Work out the finished part from the listing and answer in its coordinate system (mm). Face numbers are marked on the shaded views. A direction names the side the tool comes from. Give positions to 0.01 mm unless a question says otherwise; leave off trailing zeros. Write each loop counter-clockwise with the first axis right and the second up, starting at its lowest first coordinate (ties: lowest second). Pieces come first, ordered by that corner, then holes. Notation, with made-up numbers: (25, 75) -> (76, 75) arc R23 ccw to (76, 111) -> close; hole circle Ø4 at (-29.75, 47.5). An arc over 180 degrees is marked (long way). Use a Markdown table: item, result. Add a question column.
Q1. Each of these flat-tipped pins is pushed along its axis until it touches: pin 1 Ø2.5 at (x, y) = (0.5, -5) entering from +Z; pin 2 Ø1.5 at (y, z) = (14, -2.5) entering from -X; pin 3 Ø0.8 at (y, z) = (-5, -1.5) entering from +X. Where does it stop, or does it pass through?
Q2. Section A-A, the plane y = -1.5 is taken. Give the vertices of the cut face in (x, z), plus the area to 3 significant figures.
Q3. Section B-B, the plane x = 0 is taken. Give the vertices of the cut face in (y, z), plus the area to 3 significant figures.
Q4. Section D-D, the plane y = 19.5 is taken. Give the vertices of the cut face in (x, z), plus the area to 3 significant figures.
Q5. Consider line 1 (Y direction, x = -3.5, z = -1.5); line 2 (Z direction, x = -4, y = 0.5); line 3 (Y direction, x = 0.5, z = 0.25). Determine where each line is inside the solid, lowest interval first.
Q6. For the marked faces 4, 5 and 6, determine the directions among +Z, -Z, +X, -X, +Y, -Y from which every point of the face is accessible in a straight line to the end or side of a thin tool.
Q7. Section C-C, the plane z = 0 is taken. Give the vertices of the cut face in (x, y).
Q8. For a pull along Y with two mould halves and no side action, classify the marked faces 1, 2 and 3 as pulls with the +Y half, pulls with the -Y half, needs draft (parallel to the pull), parting line crosses it, or undercut.
from build123d import *

# Parameters (mm, degrees)
ESQUISSE3_W        = 3
ESQUISSE3_H        = 1
BOSS_EXTRU_1_DEPTH = 8


with BuildPart() as part:
    # Esquisse1 → Révolution1 (revolve)
    with BuildSketch(Plane.XY):
        Polygon((0, 0), (-5, 0), (-5, 13), (-6, 13), (-6, 18), (-3, 18), (-3, 20.5), (0, 20.5), align=None)
    revolve(axis=Axis((0, 0, 0), (0, 1, 0)))

    # Esquisse2 → Révolution2 (revolve)
    with BuildSketch(Plane.XY):
        with BuildLine():
            Line((0, 20.5), (-5, 20.5))
            Line((-5, 20.5), (-5, 22.5))
            ThreePointArc((-5, 22.5), (-4.707106781, 23.207106781), (-4, 23.5))
            Line((-4, 23.5), (0, 23.5))
            Line((0, 23.5), (0, 20.5))
        make_face()
    revolve(axis=Axis((0, 20.5, 0), (0, 1, 0)))

    # Esquisse3 → Boss.-Extru.1 (add)
    with BuildSketch(Plane.XZ):
        with Locations((0, -1.5)):
            Rectangle(ESQUISSE3_W, ESQUISSE3_H)
        with Locations((0, 1.5)):
            Rectangle(ESQUISSE3_W, ESQUISSE3_H)
    extrude(amount=BOSS_EXTRU_1_DEPTH)


solid = part.part
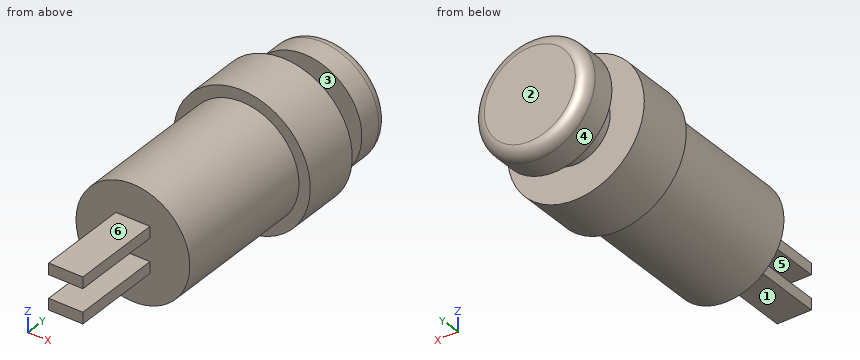
Result set:
| question | item | result |
|---|---|---|
| 1 | pin 1 | stops at z = 2 |
| 1 | pin 2 | stops at x = -5.74 |
| 1 | pin 3 | stops at x = 1.5 |
| 2 | outline | (-1.5, -2) -> (1.5, -2) -> (1.5, -1) -> (-1.5, -1) -> close; (-1.5, 1) -> (1.5, 1) -> (1.5, 2) -> (-1.5, 2) -> close |
| 2 | area | 6.00 mm2 |
| 3 | outline | (-8, -2) -> (0, -2) -> (0, -5) -> (13, -5) -> (13, -6) -> (18, -6) -> (18, -3) -> (20.5, -3) -> (20.5, -5) -> (22.5, -5) arc R1 ccw to (23.5, -4) -> (23.5, 4) arc R1 ccw to (22.5, 5) -> (20.5, 5) -> (20.5, 3) -> (18, 3) -> (18, 6) -> (13, 6) -> (13, 5) -> (0, 5) -> (0, 2) -> (-8, 2) -> (-8, 1) -> (0, 1) -> (0, -1) -> (-8, -1) -> close |
| 3 | area | 251 mm2 |
| 4 | outline | circle Ø6 at (0, 0) |
| 4 | area | 28.3 mm2 |
| 5 | line 1 | y = 0 to 18, 20.5 to 23.5 |
| 5 | line 2 | z = -3 to 3 |
| 5 | line 3 | y = 0 to 23.5 |
| 6 | face 4 | +Y |
| 6 | face 5 | +X, -X, -Y |
| 6 | face 6 | +Z, +X, -X, -Y |
| 7 | outline | (-6, 13) -> (-5, 13) -> (-5, 0) -> (5, 0) -> (5, 13) -> (6, 13) -> (6, 18) -> (3, 18) -> (3, 20.5) -> (5, 20.5) -> (5, 22.5) arc R1 ccw to (4, 23.5) -> (-4, 23.5) arc R1 ccw to (-5, 22.5) -> (-5, 20.5) -> (-3, 20.5) -> (-3, 18) -> (-6, 18) -> close |
| 8 | face 1 | needs draft |
| 8 | face 2 | pulls with the +Y half |
| 8 | face 3 | undercut |
